```python
from build123d import *

# Parameters (mm, degrees)
SKETCH1_R           = 1.35
SKETCH1_R_2         = 3
BOSS_EXTRUDE1_DEPTH = 10
SKETCH9_R           = 3
BOSS_EXTRUDE2_DEPTH = 3
SKETCH10_W          = 38
SKETCH10_H          = 6
CUT_EXTRUDE3_DEPTH  = 8
FILLET3_R           = 15
FILLET4_R           = 1.2
CUT_EXTRUDE4_REACH  = 137.355
CUT_EXTRUDE5_DEPTH  = 56
SKETCH13_R          = 3
SKETCH13_R_2        = 1.6
BOSS_EXTRUDE3_DEPTH = 5
FILLET5_R           = 1.2
CUT_EXTRUDE6_DEPTH  = 160.5
SKETCH15_W          = 146.140561772
SKETCH15_H          = 38.947987949
CUT_EXTRUDE7_DEPTH  = 13


with BuildPart() as part:
    # Sketch1 → Boss-Extrude1 (new body)
    with BuildSketch(Plane(origin=(0, 0, 0), x_dir=(1, 0, 0), z_dir=(0, 1, 0))):
        with BuildLine():
            Line((0, 14), (120, 14))
            Line((120, 14), (120, -14))
            Line((120, -14), (0, -14))
            ThreePointArc((0, -14), (-14, 0), (0, 14))
        make_face()
        with Locations(Location((85, 9, 0), (0, 0, 270))):
            Circle(SKETCH1_R, mode=Mode.SUBTRACT)
        with Locations(Location((60, 9, 0), (0, 0, 270))):
            Circle(SKETCH1_R, mode=Mode.SUBTRACT)
        with Locations(Location((110, 9, 0), (0, 0, 270))):
            Circle(SKETCH1_R, mode=Mode.SUBTRACT)
        with Locations(Location((10, 9, 0), (0, 0, 90))):
            Circle(SKETCH1_R, mode=Mode.SUBTRACT)
        with Locations(Location((35, 9, 0), (0, 0, 90))):
            Circle(SKETCH1_R, mode=Mode.SUBTRACT)
        with Locations(Location((0, 0, 0), (0, 0, 270))):
            Circle(SKETCH1_R_2, mode=Mode.SUBTRACT)
        with BuildLine():
            Line((70, -8.5), (50, -8.5))
            ThreePointArc((50, -8.5), (47.5, -6), (50, -3.5))
            Line((50, -3.5), (70, -3.5))
            ThreePointArc((70, -3.5), (72.5, -6), (70, -8.5))
        make_face(mode=Mode.SUBTRACT)
        with BuildLine():
            Line((90, -3.5), (110, -3.5))
            ThreePointArc((110, -3.5), (112.5, -6), (110, -8.5))
            Line((110, -8.5), (90, -8.5))
            ThreePointArc((90, -8.5), (87.5, -6), (90, -3.5))
        make_face(mode=Mode.SUBTRACT)
    extrude(amount=BOSS_EXTRUDE1_DEPTH)

    # Sketch9 → Boss-Extrude2 (add)
    with BuildSketch(Plane(origin=(0, 10, 0), x_dir=(1, 0, 0), z_dir=(0, 1, 0))):
        with BuildLine():
            Line((0, 14), (24.5, 14))
            Line((24.5, 14), (24.5, -14))
            Line((24.5, -14), (0, -14))
            ThreePointArc((0, -14), (-14, 0), (0, 14))
        make_face()
        with Locations(Location((0, 0, 0), (0, 0, 270))):
            Circle(SKETCH9_R, mode=Mode.SUBTRACT)
    extrude(amount=BOSS_EXTRUDE2_DEPTH)

    # Sketch10 → Cut-Extrude3 (cut)
    with BuildSketch(Plane(origin=(0, 13, 0), x_dir=(1, 0, 0), z_dir=(0, 1, 0))):
        with Locations((19, 0)):
            Rectangle(SKETCH10_W, SKETCH10_H)
    extrude(amount=-CUT_EXTRUDE3_DEPTH, mode=Mode.SUBTRACT)

    # Fillet3
    fillet3_edges = [part.edges().sort_by_distance(p)[0] for p in [
        (120, 5, -14),
    ]]
    fillet(fillet3_edges, radius=FILLET3_R)

    # Fillet4
    # the kernel refuses this fillet: 1.2 mm, written as the material it adds along each edge
    with BuildSketch(Plane(origin=(-3, 5, -3), x_dir=(0, 1, 0), z_dir=(1, 0, 0))) as fillet4_piece_1_section:
        with BuildLine():
            CenterArc((FILLET4_R, FILLET4_R), FILLET4_R, 180, 90)
            Line((0, FILLET4_R), (0, 0))
            Line((0, 0), (FILLET4_R, 0))
        make_face()
    fillet4_piece_1 = extrude(amount=44, mode=Mode.PRIVATE)
    fillet4_piece_1 = fillet4_piece_1 - Plane(origin=(0, 5.276873311, 0), x_dir=(0, 0, 1), z_dir=(0, -1, 0)) * Cylinder(3, 93, mode=Mode.PRIVATE)
    add(fillet4_piece_1)
    with BuildSketch(Plane(origin=(41, 5, 3), x_dir=(0, 1, 0), z_dir=(-1, 0, 0))) as fillet4_piece_2_section:
        with BuildLine():
            CenterArc((FILLET4_R, FILLET4_R), FILLET4_R, 180, 90)
            Line((0, FILLET4_R), (0, 0))
            Line((0, 0), (FILLET4_R, 0))
        make_face()
    fillet4_piece_2 = extrude(amount=44, mode=Mode.PRIVATE)
    fillet4_piece_2 = fillet4_piece_2 - Plane(origin=(0, 5.276873499, 0), x_dir=(0, 0, 1), z_dir=(0, -1, 0)) * Cylinder(3, 93, mode=Mode.PRIVATE)
    add(fillet4_piece_2)

    # Cut-Extrude4: up to this face of the body (flat: up to its plane)
    cut_extrude4_end = Plane(part.part.faces().sort_by_distance((24.5, 11.5, 8.5))[0])
    # Sketch4 → Cut-Extrude4 (cut, up to the picked face)
    with BuildSketch(Plane(origin=(120, 0, 0), x_dir=(0, 0, -1), z_dir=(1, 0, 0)), mode=Mode.PRIVATE) as cut_extrude4_sk1:
        Polygon((-14, 10), (-14, 8.5), (14, 10), align=None)
    cut_extrude4_tool1 = split(extrude(cut_extrude4_sk1.sketch, amount=-CUT_EXTRUDE4_REACH, mode=Mode.PRIVATE), bisect_by=cut_extrude4_end, keep=Keep.BOTH, mode=Mode.PRIVATE)
    add(cut_extrude4_tool1.solids().sort_by(Axis((120, 9.5, 4.666667), (-1, 0, 0)))[0], mode=Mode.SUBTRACT)

    # Sketch11 → Cut-Extrude5 (cut)
    with BuildSketch(Plane(origin=(0, 0, -14), x_dir=(-1, 0, 0), z_dir=(0, 0, -1))):
        with BuildLine():
            add(Edge.make_bspline(
                [(-120, 5.696428571), (-112.075751897, 0.845176506), (-105, 0)],
                knots=[0, 0, 0, 0.27358728, 0.27358728, 0.27358728], degree=2))
            Line((-105, 0), (-120, 0))
            Line((-120, 0), (-120, 5.696428571))
        make_face()
    extrude(amount=-CUT_EXTRUDE5_DEPTH, mode=Mode.SUBTRACT)

    # Sketch13 → Boss-Extrude3 (add)
    with BuildSketch(Plane.XZ):
        Circle(SKETCH13_R)
        with Locations(Location((0, 0, 0), (0, 0, 270))):
            Circle(SKETCH13_R_2, mode=Mode.SUBTRACT)
    extrude(amount=-BOSS_EXTRUDE3_DEPTH)

    # Fillet5
    fillet5_edges = [part.edges().sort_by_distance(p)[0] for p in [
        (-14, 13, 0),
        (12.25, 13, 14),
        (12.25, 13, -14),
    ]]
    fillet(fillet5_edges, radius=FILLET5_R)

    # Sketch14 → Cut-Extrude6 (cut)
    with BuildSketch(Plane(origin=(120, 0, 0), x_dir=(0, 0, -1), z_dir=(1, 0, 0))):
        with BuildLine():
            Line((14, 0), (11.5, 0))
            add(Edge.make_bspline(
                [(11.5, 0), (13.101323316, 0.782640841), (14, 3)],
                knots=[0, 0, 0, 0.269080741, 0.269080741, 0.269080741], degree=2))
            Line((14, 3), (14, 0))
        make_face()
    extrude(amount=-CUT_EXTRUDE6_DEPTH, mode=Mode.SUBTRACT)

    # Mirror1: part across plane


with BuildPart() as part_1:
    add(part.part)
    add(part.part.mirror(Plane.ZX.offset(13)))

    # Sketch15 → Cut-Extrude7 (cut)
    with BuildSketch(Plane.XZ):
        with Locations((46.929719114, -5.473993975)):
            Rectangle(SKETCH15_W, SKETCH15_H)
    extrude(amount=-CUT_EXTRUDE7_DEPTH, mode=Mode.SUBTRACT)


solid = part_1.part
```
Model file for the job. Use its own axes, mm. A direction names the side the tool comes from. Round coordinates to 2 decimals unless told otherwise and drop trailing zeros. One line per item, written item: value.
(1) Two-plate mould, pull along Z, no slides. Class faces 5 (the flat face through (60, 22, 3.5)), 6 (the flat face through (24.5, 15, 8)), 7 (the flat face through (52, 20, -14)): pulls with the +Z half, pulls with the -Z half, needs draft (parallel to the pull), parting line crosses it, or undercut.
Values follow:
face 5: undercut
face 6: needs draft
face 7: pulls with the -Z half
(2) Wall check: probe 1 along Z at (x, y) = (60, 20.75); probe 2 along Z at (x, y) = (95.5, 20.5); probe 3 along X at (y, z) = (21.25, -9). Give the ranges that are in metal, low to high.
Values follow:
probe 1: z = -14 to -10.35, -7.65 to 3.5, 8.5 to 14
probe 2: z = -14 to 3.5, 8.5 to 14
probe 3: x = -10.72 to 8.65, 11.35 to 33.65, 36.35 to 58.65, 61.35 to 83.65, 86.35 to 108.65, 111.35 to 116.18
(3) 3-axis set-ups, long thin cutter, end or side, ignore diameter. For faces 1 (the flat face through (100, 22, 8.5)), 2 (the flat face through (10, 16, -9)), 3 (the flat face through (17, 21, 0)), 4 (the flat face through (72.92, 16.76, 0.2)): which of +Z, -Z, +X, -X, +Y, -Y reach the whole face in a straight line?
Values follow:
face 1: +Y, -Y
face 2: +Y
face 3: -Y
face 4: +Z, +X, -Y
(4) Cut at A-A, the plane z = 6. Give the number of separate pieces and of enclosed holes in the cut face, plus the area to 3 significant figures.
Values follow:
separate pieces: 3
enclosed holes: 0
area: 861 mm²
(5) Drop flat-ended pins along their axis: P1, Ø4, axis at x = 102.5, z = 7.5, coming from the -Y side; P2, Ø1.1, axis at y = 15, z = -6.5, coming from the +X side; P3, Ø2.5, axis at x = 110, z = -9, coming from the +Y side; P4, Ø5, axis at y = 24, z = -9.5, coming from the -X side. Give the stop position or say it passes through.
Values follow:
P1: stops at y = 17.21
P2: stops at x = 24.5
P3: passes through
P4: stops at x = -12.12
